Read the model definition and answer for the solid it produces. Units are mm, in the model's axes. Face numbers are marked on the shaded views. A direction names the side the tool comes from. Round coordinates to 2 decimals unless told otherwise and drop trailing zeros. Write each loop counter-clockwise with the first axis right and the second up, starting at its lowest first coordinate (ties: lowest second). Pieces come first, ordered by that corner, then holes. Notation, with made-up numbers: (0, -32.5) - (52, -32.5) arc R24 ccw to (52, 0.5) - close; hole circle Ø1 at (-37, 88). An arc over 180 degrees is marked (long way). Answer as CSV lines item,"result". Start each with the question number.
1) Which of the six approach directions +Z, -Z, +X, -X, +Y, -Y give full straight-line access (tool end or side, diameter ignored) to the marked faces 1, 2 and 3?
2) For a pull along Z with two mould halves and no side action, classify the marked faces 4, 5, 6 and 7 as +Z half, -Z half, draft (parallel to the pull), parting line (faces both ways), or undercut.
3) Each of these flat-tipped pins is pushed along its axis until it touches: pin 1 (3 mm diameter, centred on x = 0, z = -13.5, fed in from -Y); pin 2 (9.5 mm diameter, centred on x = 0, z = 0, fed in from -Y); pin 3 (1.5 mm diameter, centred on x = 14, z = -12, fed in from +Y). Where does it stop, or does it pass through?
4) Find section A-A on x = 0. Determine the outline of the cut face in (y, z).
5) Find section B-B on z = 0. Determine the outline of the cut face in (x, y).
6) Find section C-C on y = 8. Determine the outline of the cut face in (x, z), then the cut area to 3 significant figures.
7) Consider line 1 along X through (y, z) = (-5.5, 0); line 2 along X through (y, z) = (-2.7, 0); line 3 along Z through (x, y) = (7, 3.5). Determine where each line is inside the solid, lowest interval first.
8) Find section D-D on z = 13.5. Determine the outline of the cut face in (x, y).
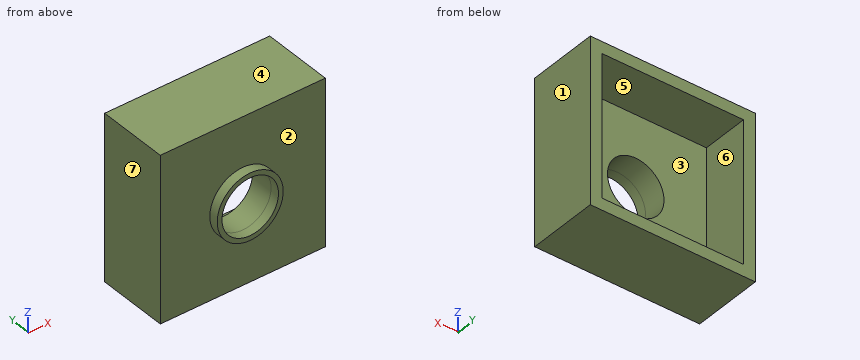
from build123d import *

# Parameters (mm, degrees)
SKETCH1_W           = 35
SKETCH1_H           = 35
SKETCH1_W_2         = 30
SKETCH1_H_2         = 30
BOSS_EXTRUDE1_DEPTH = 10
SKETCH4_W           = 35
SKETCH4_H           = 35
BOSS_EXTRUDE2_DEPTH = 5
SKETCH5_R           = 6
CUT_EXTRUDE1_DEPTH  = 29.939592257
SKETCH6_R           = 7
SKETCH6_R_2         = 6
BOSS_EXTRUDE3_DEPTH = 2


with BuildPart() as part:
    # Sketch1 → Boss-Extrude1 (new body)
    with BuildSketch(Plane(origin=(0, 0, 0), x_dir=(1, 0, 0), z_dir=(0, 1, 0))):
        Rectangle(SKETCH1_W, SKETCH1_H)
        Rectangle(SKETCH1_W_2, SKETCH1_H_2, mode=Mode.SUBTRACT)
    extrude(amount=BOSS_EXTRUDE1_DEPTH)

    # Sketch4 → Boss-Extrude2 (add)
    with BuildSketch(Plane.XZ):
        Rectangle(SKETCH4_W, SKETCH4_H)
    extrude(amount=BOSS_EXTRUDE2_DEPTH)

    # Sketch5 → Cut-Extrude1 (cut, through all)
    with BuildSketch(Plane.XZ.offset(5)):
        with Locations(Location((0, 0, 0), (0, 0, 270))):
            Circle(SKETCH5_R)
    extrude(amount=-CUT_EXTRUDE1_DEPTH, mode=Mode.SUBTRACT)

    # Sketch6 → Boss-Extrude3 (add)
    with BuildSketch(Plane(origin=(0, -5, 0), x_dir=(-1, 0, 0), z_dir=(0, -1, 0))):
        with Locations(Location((0, 0, 0), (0, 0, 270))):
            Circle(SKETCH6_R)
        with Locations(Location((0, 0, 0), (0, 0, 90))):
            Circle(SKETCH6_R_2, mode=Mode.SUBTRACT)
    extrude(amount=BOSS_EXTRUDE3_DEPTH)


solid = part.part
Check values:
1,face 1,"+Z, -Z, +X, +Y, -Y"
1,face 2,"-Y"
1,face 3,"+Y"
2,face 4,"+Z half"
2,face 5,"undercut"
2,face 6,"undercut"
2,face 7,"draft"
3,pin 1,"stops at y = -5"
3,pin 2,"passes through"
3,pin 3,"stops at y = 0"
4,outline,"(-7, -7) - (-5, -7) - (-5, -17.5) - (10, -17.5) - (10, -15) - (0, -15) - (0, -6) - (-7, -6) - close; (-7, 6) - (0, 6) - (0, 15) - (10, 15) - (10, 17.5) - (-5, 17.5) - (-5, 7) - (-7, 7) - close"
5,outline,"(-17.5, -5) - (-7, -5) - (-7, -7) - (-6, -7) - (-6, 0) - (-15, 0) - (-15, 10) - (-17.5, 10) - close; (6, -7) - (7, -7) - (7, -5) - (17.5, -5) - (17.5, 10) - (15, 10) - (15, 0) - (6, 0) - close"
6,outline,"(-17.5, -17.5) - (17.5, -17.5) - (17.5, 17.5) - (-17.5, 17.5) - close; hole (-15, -15) - (15, -15) - (15, 15) - (-15, 15) - close"
6,area,"325 mm^2"
7,line 1,"x = -7 to -6, 6 to 7"
7,line 2,"x = -17.5 to -6, 6 to 17.5"
7,line 3,"z = -17.5 to -15, 15 to 17.5"
8,outline,"(-17.5, -5) - (17.5, -5) - (17.5, 10) - (15, 10) - (15, 0) - (-15, 0) - (-15, 10) - (-17.5, 10) - close"
